The listing builds one solid part. Answer for the finished solid, in the listing's coordinates (mm). A direction names the side the tool comes from. Coordinates: 2 decimals unless noted, no trailing zeros. Order: outer loops, then holes, each group sorted by start corner. A loop starts at its lowest first (then second) coordinate and runs counter-clockwise, first axis right, second up. Notation, with made-up numbers: (0, -27) -> (12, -27) arc R21 cw to (12, -4) -> close; hole circle Ø8 at (-24, -32.75). An arc over 180 degrees is marked (long way). Answer in a Markdown table with one row per item.
```python
from build123d import *

# Parameters (mm, degrees)
BOSS_EXTRUDE1_DEPTH = 1.25
SKETCH2_W           = 122.3
SKETCH2_H           = 31
CUT_EXTRUDE1_DEPTH  = 0.6


with BuildPart() as part:
    # Sketch1 → Boss-Extrude1 (new body)
    with BuildSketch(Plane(origin=(0, 0, 0), x_dir=(1, 0, 0), z_dir=(0, 1, 0))):
        Polygon((8, 0), (53, 0), (53, 2), (56, 2), (56, 0), (74.3, 0), (74.3, 2), (77.3, 2), (77.3, 0), (127.3, 0), (127.3, 2), (132.3, 2), (132.3, 39), (127.3, 39), (127.3, 41), (77.3, 41), (77.3, 39), (74.3, 39), (74.3, 41), (56, 41), (56, 39), (53, 39), (53, 41), (8, 41), (8, 39), (5, 39), (5, 41), (0, 41), (0, 0), (5, 0), (5, 2), (8, 2), align=None)
    extrude(amount=BOSS_EXTRUDE1_DEPTH)

    # Sketch2 → Cut-Extrude1 (cut)
    with BuildSketch(Plane(origin=(0, 1.25, 0), x_dir=(1, 0, 0), z_dir=(0, 1, 0))):
        with Locations((66.15, 20.5)):
            Rectangle(SKETCH2_W, SKETCH2_H)
    extrude(amount=-CUT_EXTRUDE1_DEPTH, mode=Mode.SUBTRACT)


solid = part.part
```
(1) A cutting plane is placed at B-B, the plane z = -24.5. Determine the outline of the cut face in (x, y).
Check values:
| item | result |
|---|---|
| outline | (0, 0) -> (132.3, 0) -> (132.3, 1.25) -> (127.3, 1.25) -> (127.3, 0.65) -> (5, 0.65) -> (5, 1.25) -> (0, 1.25) -> close |
(2) Which of the six approach directions +Z, -Z, +X, -X, +Y, -Y give full straight-line access (tool end or side, diameter ignored) to faces 1 (the flat face through (65, 0.65, -21)), 2 (the flat face through (65, 0, -21))?
Check values:
| item | result |
|---|---|
| face 1 | +Y |
| face 2 | +Z, -Z, +X, -X, -Y |
(3) A cutting plane is placed at A-A, the plane x = 102. Determine the outline of the cut face in (y, z), then the cut area to 4 significant figures.
Check values:
| item | result |
|---|---|
| outline | (0, -41) -> (1.25, -41) -> (1.25, -36) -> (0.65, -36) -> (0.65, -5) -> (1.25, -5) -> (1.25, 0) -> (0, 0) -> close |
| area | 32.65 mm² |
(4) Flat-ended cylindrical pins translate along their axes: pin 1 (0.6 mm diameter, centred on y = 0.5, z = -39.5, fed in from -X); pin 2 (15.5 mm diameter, centred on x = 59, z = -25.5, fed in from +Y). Find the tip coordinate at first contact, or state that the pin passes through.
Check values:
| item | result |
|---|---|
| pin 1 | x = 0 |
| pin 2 | y = 0.65 |
(5) Find the intervals of material crossed by line 1 along Z through (x, y) = (64, 0.8); line 2 along X through (y, z) = (0.85, -8.5); line 3 along Y through (x, z) = (49.5, -11), in increasing order. Write a range as from..to.
Check values:
| item | result |
|---|---|
| line 1 | -41..-36, -5..0 |
| line 2 | 0..5, 127.3..132.3 |
| line 3 | 0..0.65 |
